Design review of the part built by this model. Coordinates are the model's own, in mm. Give positions to 0.01 mm unless a question says otherwise; leave off trailing zeros. Loops run counter-clockwise (first coordinate to the right, second up) from the corner with the lowest first, then second, coordinate; pieces in that order, holes last. Notation, with made-up numbers: (-7, 49) -> (11, 49) arc R24 ccw to (11, 84) -> close; hole circle Ø11 at (86.5, 39.25). An arc over 180 degrees is marked (long way). Answer in a Markdown table with one row per item. Add a question column.
(1) For pin 1 (4 mm diameter, centred on y = 361, z = 3.5, fed in from +X) (3 decimals); pin 2 (1.5 mm diameter, centred on x = 197, z = 9.5, fed in from +Y), all flat-tipped, find the tip position at first contact; note any pin that passes through.
(2) For line 1 (Y direction, x = 250, z = 10); line 2 (X direction, y = 38, z = 17.5); line 3 (X direction, y = -252, z = 15.75), list the stretches that pass through material, from the lowest coordinate up.
(3) Consider section B-B on z = 5.25. Write out the cut boundary in (x, y), then the cut area to 3 significant figures.
(4) Consider section A-A on y = 222. Write out the cut boundary in (x, z).
(5) Consider section C-C on x = 393.5. Write out the cut boundary in (y, z).
Autodesk Inventor part; units mm, degrees
ref_plane "YZ Plane" through (0, 0, 0) normal (1, 0, 0) x (0, 1, 0)
ref_plane "XZ Plane" through (0, 0, 0) normal (0, 1, 0) x (-1, 0, 0)
ref_plane "XY Plane" through (0, 0, 0) normal (0, 0, 1) x (1, 0, 0)
sketch "Sketch1" plane through (0, 0, 0) normal (0, 0, 1) x (1, 0, 0)
  line L0 (457.2, -406.4) -> (457.2, -609.6)
  line L1 (457.2, -609.6) -> (-457.2, -609.6)
  line L2 (-457.2, -609.6) -> (-457.2, 609.6)
  line L3 (-457.2, 609.6) -> (-330.2, 609.6)
  line L4 (762.0015, 0.0045) -> (-761.9985, -0.0045) construction
  line L5 (457.2, -609.6) -> (-457.2, 609.6) construction
  line L6 (457.2, -406.4) -> (-330.2, 609.6)
  point P0 (0, 0)
  dimension "d0" = 681.5582
  dimension "d1" = 914.4
  dimension "d2" = 203.2
  dimension "d3" = 127
  dimension "d4" = 1219.2
extrude "Extrusion1" add sketch "Sketch1" along normal blind 25.4
properties part number "stock wall triangl"
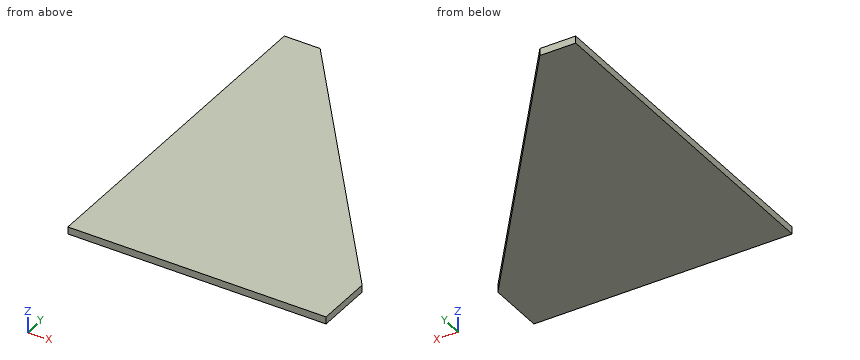
Values follow:
| question | item | result |
|---|---|---|
| 1 | pin 1 | x = -135.985 |
| 1 | pin 2 | y = -69.69 |
| 2 | line 1 | -609.6 to -139.05 |
| 2 | line 2 | -457.2 to 112.79 |
| 2 | line 3 | -457.2 to 337.54 |
| 3 | outline | (-457.2, -609.6) -> (457.2, -609.6) -> (457.2, -406.4) -> (-330.2, 609.6) -> (-457.2, 609.6) -> close |
| 3 | area | 715,000 mm2 |
| 4 | outline | (-457.2, 0) -> (-29.81, 0) -> (-29.81, 25.4) -> (-457.2, 25.4) -> close |
| 5 | outline | (-609.6, 0) -> (-324.21, 0) -> (-324.21, 25.4) -> (-609.6, 25.4) -> close |
